from build123d import *

# Parameters (mm, degrees)
BOSS_EXTRUDE1_DEPTH            = 32
SKETCH2_R                      = 6
CUT_EXTRUDE1_DEPTH             = 22
SKETCH3_R                      = 5
CUT_EXTRUDE2_DEPTH             = 4
CUT_EXTRUDE3_REACH             = 43
SKETCH4_R                      = 3
CUT_EXTRUDE3_DIRECTION_2_DEPTH = 5.0000001
SKETCH5_R                      = 3
CUT_EXTRUDE4_DEPTH             = 16


with BuildPart() as part:
    # Sketch1 → Boss-Extrude1 (new body)
    with BuildSketch(Plane.XY):
        Polygon((40, 0), (64, 0), (64, 36), (0, 36), (0, 0), (24, 0), (24, -9), (40, -9), align=None)
    extrude(amount=BOSS_EXTRUDE1_DEPTH)

    # Sketch2 → Cut-Extrude1 (cut)
    with BuildSketch(Plane.XY.offset(32)):
        with BuildLine():
            Line((0, 36), (0, 10))
            Line((0, 10), (3, 10))
            ThreePointArc((3, 10), (4.341640786, 10.316718427), (5.4, 11.2))
            Line((5.4, 11.2), (19.2, 29.6))
            ThreePointArc((19.2, 29.6), (24.844582472, 34.310835056), (32, 36))
            Line((32, 36), (0, 36))
        make_face()
        with BuildLine():
            Line((64, 36), (32, 36))
            ThreePointArc((32, 36), (39.155417528, 34.310835056), (44.8, 29.6))
            Line((44.8, 29.6), (58.6, 11.2))
            ThreePointArc((58.6, 11.2), (59.658359214, 10.316718427), (61, 10))
            Line((61, 10), (64, 10))
            Line((64, 10), (64, 36))
        make_face()
        with Locations((32, 20)):
            Circle(SKETCH2_R)
    extrude(amount=-CUT_EXTRUDE1_DEPTH, mode=Mode.SUBTRACT)

    # Sketch3 → Cut-Extrude2 (cut)
    with BuildSketch(Plane(origin=(0, 36, 0), x_dir=(1, 0, 0), z_dir=(0, 1, 0))):
        with Locations((32, -20)):
            Circle(SKETCH3_R)
    extrude(amount=-CUT_EXTRUDE2_DEPTH, mode=Mode.SUBTRACT)

    # Sketch4 → Cut-Extrude3 (cut, up to next)
    with BuildSketch(Plane(origin=(0, 32, 0), x_dir=(1, 0, 0), z_dir=(0, 1, 0)), mode=Mode.PRIVATE) as cut_extrude3_sk1:
        with Locations((32, -20)):
            Circle(SKETCH4_R)
    cut_extrude3_tool1 = extrude(cut_extrude3_sk1.sketch, amount=-CUT_EXTRUDE3_REACH, mode=Mode.PRIVATE) & part.part
    add(cut_extrude3_tool1.solids().sort_by_distance((32, 32, 20))[0], mode=Mode.SUBTRACT)

    # Sketch4 → Cut-Extrude3 direction 2 (cut)
    with BuildSketch(Plane(origin=(0, 32, 0), x_dir=(1, 0, 0), z_dir=(0, 1, 0))):
        with Locations((32, -20)):
            Circle(SKETCH4_R)
    extrude(amount=CUT_EXTRUDE3_DIRECTION_2_DEPTH, mode=Mode.SUBTRACT)

    # Sketch5 → Cut-Extrude4 (cut)
    with BuildSketch(Plane.XZ.offset(9)):
        with Locations((32, 24)):
            Circle(SKETCH5_R)
        with Locations((32, 8)):
            Circle(SKETCH5_R)
    extrude(amount=-CUT_EXTRUDE4_DEPTH, mode=Mode.SUBTRACT)


solid = part.part
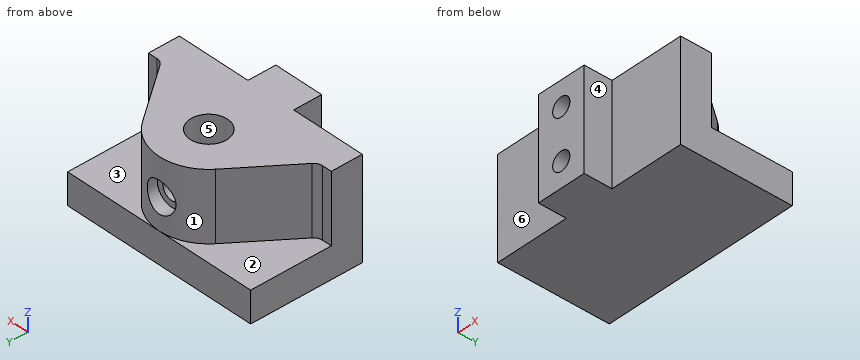
Source: CAD feature listing. Evaluate the final solid. Frame: model axes, mm. Face numbers are marked on the shaded views. A direction names the side the tool comes from. Round coordinates to 2 decimals unless told otherwise and drop trailing zeros. Write each loop counter-clockwise with the first axis right and the second up, starting at its lowest first coordinate (ties: lowest second). Pieces come first, ordered by that corner, then holes. Notation, with made-up numbers: (28.25, 0) - (49.25, 0) arc R36 ccw to (49.25, 37) - close; hole circle Ø9 at (12.25, -13). An arc over 180 degrees is marked (long way). Use CSV: the item, a comma, the result in double quotes. Start each with the question number.
(1) Mould query, pull axis Y, two halves, no side actions, for the marked faces 4, 5 and 6. Classes: pulls with the +Y half, pulls with the -Y half, needs draft (parallel to the pull), parting line crosses it, or undercut.
(2) First-contact query: pin 1 Ø1.5 at (y, z) = (14, 22.5) entering from +X; pin 2 Ø3.5 at (x, z) = (32, 8) entering from -Y; pin 3 Ø2.5 at (x, z) = (62, 15.5) entering from +Y. Flat tips, straight axial feed; report the tip coordinate or a pass-through.
(3) Cut plane B-B, the plane y = 3. Return loops of the section in (x, z).
(4) Cut plane A-A, the plane z = 12.5. Return loops of the section in (x, y).
(5) Cut plane D-D, the plane x = 7.5. Return loops of the section in (y, z).
(6) Material intervals for probe 1 along Z at (x, y) = (32, -0.5); probe 2 along Z at (x, y) = (32, 33.1); probe 3 along Z at (x, y) = (32, 27.25), sorted ascending. Write a range as [from, to].
(7) Set-up query: the marked faces 1, 2 and 3. Return all of +Z, -Z, +X, -X, +Y, -Y with unobstructed straight access to the full face (end or side cutting, diameter ignored); none if empty.
(8) Cut plane C-C, the plane z = 8. Return loops of the section in (x, y), and give its area (3 significant figures).
Geometry says:
1,face 4,"needs draft"
1,face 5,"undercut"
1,face 6,"pulls with the -Y half"
2,pin 1,"x = 57.06"
2,pin 2,"y = 7"
2,pin 3,"y = 10.01"
3,outline,"(0, 0) - (64, 0) - (64, 32) - (0, 32) - close; hole circle Ø6 at (32, 8); hole circle Ø6 at (32, 24)"
4,outline,"(0, 0) - (24, 0) - (24, -9) - (40, -9) - (40, 0) - (64, 0) - (64, 10) - (61, 10) arc R3 cw to (58.6, 11.2) - (44.8, 29.6) arc R16 ccw to (19.2, 29.6) - (5.4, 11.2) arc R3 cw to (3, 10) - (0, 10) - close; hole circle Ø12 at (32, 20)"
5,outline,"(0, 0) - (36, 0) - (36, 10) - (14, 10) - (14, 32) - (0, 32) - close"
6,probe 1,"[0, 5], [11, 21], [27, 32]"
6,probe 2,"[0, 15], [25, 32]"
6,probe 3,"[0, 17], [23, 32]"
7,face 1,"+Z, +Y"
7,face 2,"+Z, -X, +Y"
7,face 3,"+Z, +X, +Y"
8,outline,"(0, 0) - (24, 0) - (24, -9) - (29, -9) - (29, 7) - (35, 7) - (35, -9) - (40, -9) - (40, 0) - (64, 0) - (64, 36) - (0, 36) - close"
8,area,"2,350 mm²"
